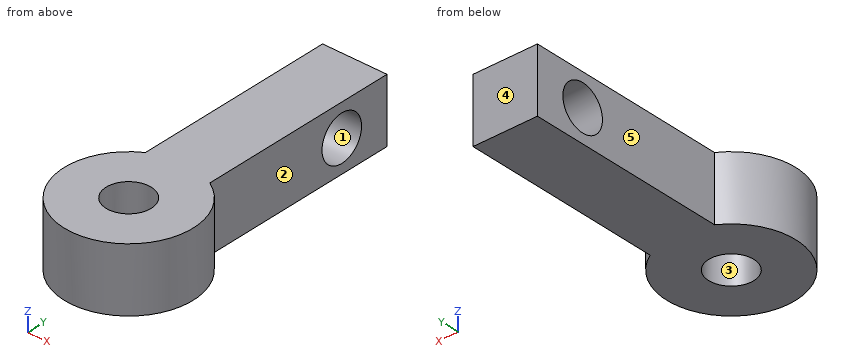
```python
from build123d import *

# Parameters (mm, degrees)
F0_R     = 1.75
F1_DEPTH = 5
F2_R     = 1.75
F3_DEPTH = 25


with BuildPart() as f1:
    # F0 (on Top) → F1 (new body)
    with BuildSketch(Plane.XY):
        with BuildLine():
            Line((2.5, -5.669873), (2.5, 10))
            Line((2.5, 10), (-2.5, 10))
            Line((-2.5, 10), (-2.5, -5.669873))
            ThreePointArc((-2.5, -5.669873), (0, -15), (2.5, -5.669873))
        make_face()
        with Locations((0, -10)):
            Circle(F0_R, mode=Mode.SUBTRACT)
    extrude(amount=F1_DEPTH)

    # F2 (on face) → F3 (cut)
    with BuildSketch(Plane(origin=(-2.5, 0, 0), x_dir=(0, -1, 0), z_dir=(-1, 0, 0))):
        with Locations((-6, 2.5)):
            Circle(F2_R)
    extrude(amount=-F3_DEPTH, mode=Mode.SUBTRACT)


solid = f1.part
```
Check sheet for the modelled part. Datum: model origin and axes. Units: mm. Face numbers are marked on the shaded views. A direction names the side the tool comes from. Coordinates: 2 decimals unless noted, no trailing zeros. Write each loop counter-clockwise with the first axis right and the second up, starting at its lowest first coordinate (ties: lowest second). Pieces come first, ordered by that corner, then holes. Notation, with made-up numbers: M 35,50.5 L 52,50.5 A7 ccw 52,63.5 Z; hole C 9,-19.75 d11. An arc over 180 degrees is marked long. Write item = value, one per line. Start each with the question number.
1. Go/stop test with flat-tipped pins: pin 1 (1.5 mm diameter, centred on y = 0.5, z = 1, fed in from +X); pin 2 (2 mm diameter, centred on y = -7.5, z = 4, fed in from +X); pin 3 (1.5 mm diameter, centred on y = 2.5, z = 3.5, fed in from -X). Record where each tip stops, or that it passes through.
2. Sectioned sample at C-C (y = -10). Record the cut outline in (x, z), then the cut area to 3 significant figures.
3. Sectioned sample at A-A (z = 2.5). Record the cut outline in (x, y).
4. Sectioned sample at D-D (y = 6). Record the cut outline in (x, z).
5. Sectioned sample at B-B (x = -0.5). Record the cut outline in (y, z).
6. Thickness scan on probe 1 along Z at (x, y) = (-1.2, 6); probe 2 along X at (y, z) = (8.5, 1.3); probe 3 along X at (y, z) = (-11.5, 0.9). Record the ranges inside material, lowest first.
7. Mould release check, pull along Y, two halves, no side actions. Record for the marked faces 3, 4 and 5: pulls with the +Y half, pulls with the -Y half, needs draft (parallel to the pull), parting line crosses it, or undercut.
8. Tool access check on the marked faces 1 and 2. Record the directions out of +Z, -Z, +X, -X, +Y, -Y that give a thin tool (end or side, any length) a straight path to the whole face; none if there is none.
The answers:
q1.pin_1 = 2.5
q1.pin_2 = 4.77
q1.pin_3 = -2.5
q2.outline = M -5,0 L -1.75,0 L -1.75,5 L -5,5 Z; M 1.75,0 L 5,0 L 5,5 L 1.75,5 Z
q2.area = 32.5 mm²
q3.outline = M -2.5,-5.67 A5 ccw long 2.5,-5.67 L 2.5,4.25 L -2.5,4.25 Z; M -2.5,7.75 L 2.5,7.75 L 2.5,10 L -2.5,10 Z; hole C 0,-10 d3.5
q4.outline = M -2.5,0 L 2.5,0 L 2.5,0.75 L -2.5,0.75 Z; M -2.5,4.25 L 2.5,4.25 L 2.5,5 L -2.5,5 Z
q5.outline = M -14.97,0 L -11.68,0 L -11.68,5 L -14.97,5 Z; M -8.32,0 L 10,0 L 10,5 L -8.32,5 Z; hole C 6,2.5 d3.5
q6.probe_1 = 0 to 0.75, 4.25 to 5
q6.probe_2 = -2.5 to 2.5
q6.probe_3 = -4.77 to -0.9, 0.9 to 4.77
q7.face_3 = undercut
q7.face_4 = pulls with the +Y half
q7.face_5 = needs draft
q8.face_1 = +X, -X
q8.face_2 = +Z, -Z, +X, +Y
